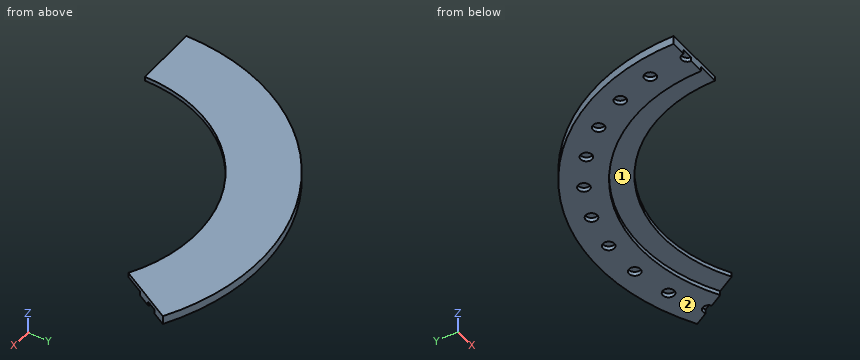
```python
from build123d import *

# Parameters (mm, degrees)
CROQUIS1_R              = 200
CROQUIS1_R_2            = 160
CROQUIS1_R_3            = 5.4
SALIENTE_EXTRUIR1_DEPTH = 4
CROQUIS2_R              = 200
CROQUIS2_R_2            = 140
SALIENTE_EXTRUIR2_DEPTH = 4
CORTAR_EXTRUIR1_DEPTH   = 10


with BuildPart() as part:
    # Croquis1 → Saliente-Extruir1 (new body)
    with BuildSketch(Plane.XY):
        Circle(CROQUIS1_R)
        Circle(CROQUIS1_R_2, mode=Mode.SUBTRACT)
        with Locations((145.623058987, 105.801345413)):
            Circle(CROQUIS1_R_3, mode=Mode.SUBTRACT)
        with Locations((164.438182376, 73.212595754)):
            Circle(CROQUIS1_R_3, mode=Mode.SUBTRACT)
        with Locations((176.066568132, 37.424104347)):
            Circle(CROQUIS1_R_3, mode=Mode.SUBTRACT)
        with Locations((180, 0)):
            Circle(CROQUIS1_R_3, mode=Mode.SUBTRACT)
        with Locations((176.066568132, -37.424104347)):
            Circle(CROQUIS1_R_3, mode=Mode.SUBTRACT)
        with Locations((164.438182376, -73.212595754)):
            Circle(CROQUIS1_R_3, mode=Mode.SUBTRACT)
        with Locations((145.623058987, -105.801345413)):
            Circle(CROQUIS1_R_3, mode=Mode.SUBTRACT)
        with Locations((120.443509145, -133.766068586)):
            Circle(CROQUIS1_R_3, mode=Mode.SUBTRACT)
        with Locations((90, -155.884572681)):
            Circle(CROQUIS1_R_3, mode=Mode.SUBTRACT)
        with Locations((55.623058987, -171.190172933)):
            Circle(CROQUIS1_R_3, mode=Mode.SUBTRACT)
        with Locations((18.815123388, -179.013941166)):
            Circle(CROQUIS1_R_3, mode=Mode.SUBTRACT)
        with Locations((-18.815123388, -179.013941166)):
            Circle(CROQUIS1_R_3, mode=Mode.SUBTRACT)
        with Locations((-55.623058987, -171.190172933)):
            Circle(CROQUIS1_R_3, mode=Mode.SUBTRACT)
        with Locations((-90, -155.884572681)):
            Circle(CROQUIS1_R_3, mode=Mode.SUBTRACT)
        with Locations((-120.443509145, -133.766068586)):
            Circle(CROQUIS1_R_3, mode=Mode.SUBTRACT)
        with Locations((-145.623058987, -105.801345413)):
            Circle(CROQUIS1_R_3, mode=Mode.SUBTRACT)
        with Locations((-164.438182376, -73.212595754)):
            Circle(CROQUIS1_R_3, mode=Mode.SUBTRACT)
        with Locations((-176.066568132, -37.424104347)):
            Circle(CROQUIS1_R_3, mode=Mode.SUBTRACT)
        with Locations((-180, 0)):
            Circle(CROQUIS1_R_3, mode=Mode.SUBTRACT)
        with Locations((-176.066568132, 37.424104347)):
            Circle(CROQUIS1_R_3, mode=Mode.SUBTRACT)
        with Locations((-164.438182376, 73.212595754)):
            Circle(CROQUIS1_R_3, mode=Mode.SUBTRACT)
        with Locations((-145.623058987, 105.801345413)):
            Circle(CROQUIS1_R_3, mode=Mode.SUBTRACT)
        with Locations((-120.443509145, 133.766068586)):
            Circle(CROQUIS1_R_3, mode=Mode.SUBTRACT)
        with Locations((-90, 155.884572681)):
            Circle(CROQUIS1_R_3, mode=Mode.SUBTRACT)
        with Locations((-55.623058987, 171.190172933)):
            Circle(CROQUIS1_R_3, mode=Mode.SUBTRACT)
        with Locations((-18.815123388, 179.013941166)):
            Circle(CROQUIS1_R_3, mode=Mode.SUBTRACT)
        with Locations((18.815123388, 179.013941166)):
            Circle(CROQUIS1_R_3, mode=Mode.SUBTRACT)
        with Locations((55.623058987, 171.190172933)):
            Circle(CROQUIS1_R_3, mode=Mode.SUBTRACT)
        with Locations((90, 155.884572681)):
            Circle(CROQUIS1_R_3, mode=Mode.SUBTRACT)
        with Locations((120.443509145, 133.766068586)):
            Circle(CROQUIS1_R_3, mode=Mode.SUBTRACT)
    extrude(amount=SALIENTE_EXTRUIR1_DEPTH)

    # Croquis2 → Saliente-Extruir2 (add)
    with BuildSketch(Plane.XY.offset(4)):
        Circle(CROQUIS2_R)
        Circle(CROQUIS2_R_2, mode=Mode.SUBTRACT)
    extrude(amount=SALIENTE_EXTRUIR2_DEPTH)

    # Croquis3 → Cortar-Extruir1 (cut)
    with BuildSketch(Plane(origin=(0, 0, 0), x_dir=(-1, 0, 0), z_dir=(0, 0, -1))):
        Polygon((-100, 173.205080757), (-166.23575866, 173.205080757), (-252.111103181, -105.177600858), (-104.783677259, -222.566833277), (177.265619424, -205.234194933), (232.312426825, -26.788589339), (200, 0), (140, 0), (-70, 121.24355653), align=None)
    extrude(amount=-CORTAR_EXTRUIR1_DEPTH, mode=Mode.SUBTRACT)


solid = part.part
```
Part model, mm, in its own coordinate system. Face numbers are marked on the shaded views. Coordinates: 2 decimals unless noted, no trailing zeros. Write each loop counter-clockwise with the first axis right and the second up, starting at its lowest first coordinate (ties: lowest second). Pieces come first, ordered by that corner, then holes.
Item 1: Mould opens along X. For the marked faces 1 and 2 say: released by +X, released by -X, zero draft, split by the parting line, or undercut.
Item 2: Slice it at B-B (y = 28). Write the cut outline in (x, z).
Item 3: Slice it at C-C (x = 39.5). Write the cut outline in (y, z).
Item 4: Slice it at A-A (z = 1.5). Count the separate pieces of the cut face and the enclosed holes in it, and give its area (3 significant figures).
Item 5: Pin check, flat tips, straight feed: pin 1 (3 mm diameter, centred on x = -173.5, y = 35, fed in from -Z); pin 2 (3 mm diameter, centred on y = 137.5, z = 5, fed in from +X); pin 3 (14 mm diameter, centred on x = 55.62, y = 171.19, fed in from -Z); pin 4 (4 mm diameter, centred on x = -126.5, z = 1, fed in from +Y). Stop position of each tip, or through.
Item 6: Slice it at D-D (x = -90). Write the cut outline in (y, z).
Item 7: Probe line 1 (X direction, y = 175.5, z = 3.5); line 2 (Z direction, x = -158, y = 17.5); line 3 (X direction, y = 145.5, z = 3.5). List the from-to ranges inside material, lowest first.
Results found:
1. face 1: undercut
1. face 2: zero draft
2. outline: (-198.03, 0) - (-157.53, 0) - (-157.53, 4) - (-137.17, 4) - (-137.17, 8) - (-198.03, 8) - close
3. outline: (134.31, 4) - (155.05, 4) - (155.05, 0) - (196.06, 0) - (196.06, 8) - (134.31, 8) - close
4. separate pieces: 1
4. enclosed holes: 9
4. area: 14,200 mm2
5. pin 1: stops at z = 4
5. pin 2: stops at x = 80.25
5. pin 3: stops at z = 0
5. pin 4: stops at y = 156.52
6. outline: (107.24, 4) - (132.29, 4) - (132.29, 0) - (150.48, 0) - (150.48, 4) - (161.28, 4) - (161.28, 0) - (178.61, 0) - (178.61, 8) - (107.24, 8) - close
7. line 1: x = -95.92 to -58.88, -52.37 to -22.92, -14.71 to 14.71, 22.92 to 52.37, 58.88 to 95.92
7. line 2: z = 4 to 8
7. line 3: x = -137.22 to -66.56, 66.56 to 84
